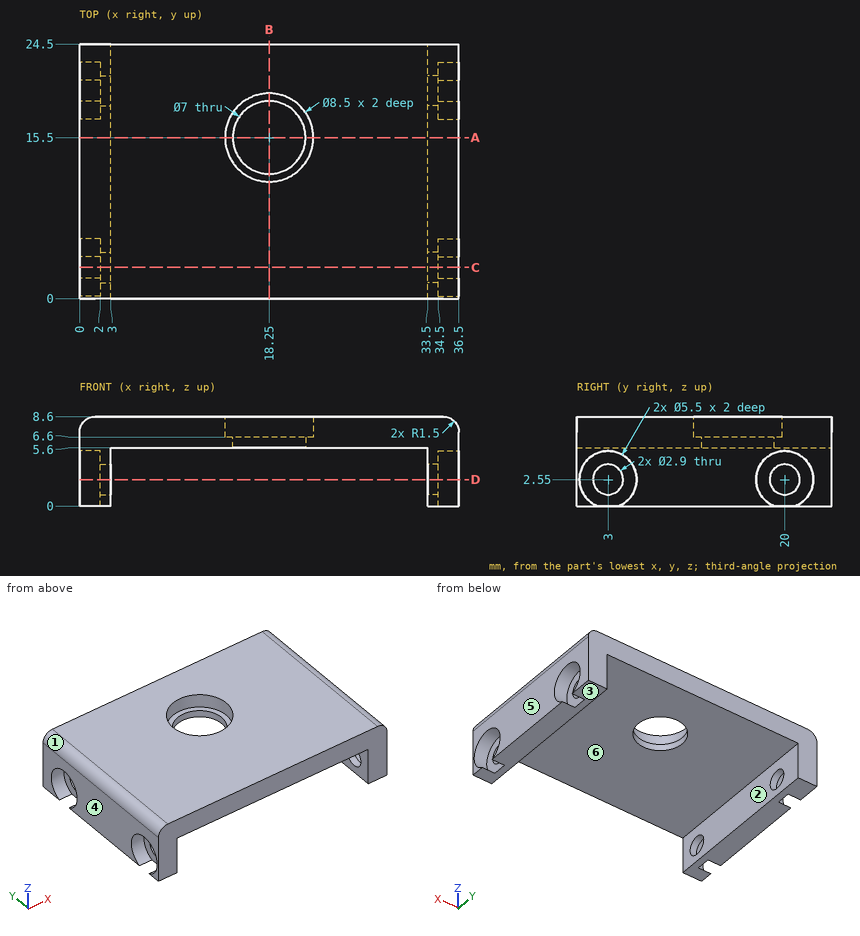
Source: three-view drawing plus pictorial views. Frame: mm from the lowest corner of the part. A direction names the side the tool comes from. Give positions to 0.01 mm unless a question says otherwise; leave off trailing zeros. Order: outer loops, then holes, each group sorted by start corner. A loop starts at its lowest first (then second) coordinate and runs counter-clockwise, first axis right, second up. Notation, with made-up numbers: M -18,-25 L 30,-25 A11 ccw 30,-19 Z; hole C 64.5,4.25 d1. An arc over 180 degrees is marked long. Return JSON: item names as keys, results as strings.
Item 1: Cut plane C-C (y = 3). Return loops of the section in (x, z), then the cut area to 3 significant figures.
Solutions:
{"outline": "M 0,5.3 L 2,5.3 L 2,4 L 3,4 L 3,5.6 L 33.5,5.6 L 33.5,4 L 34.5,4 L 34.5,5.3 L 36.5,5.3 L 36.5,7.1 A1.5 ccw 35,8.6 L 1.5,8.6 A1.5 ccw 0,7.1 Z; M 2,0 L 3,0 L 3,1.1 L 2,1.1 Z; M 33.5,0 L 34.5,0 L 34.5,1.1 L 33.5,1.1 Z", "area": "115 mm^2"}
Item 2: Cut plane A-A (y = 15.5). Return loops of the section in (x, z).
Solutions:
{"outline": "M 0,0 L 3,0 L 3,5.6 L 14.75,5.6 L 14.75,6.6 L 14,6.6 L 14,8.6 L 1.5,8.6 A1.5 ccw 0,7.1 Z; M 21.75,5.6 L 33.5,5.6 L 33.5,0 L 36.5,0 L 36.5,7.1 A1.5 ccw 35,8.6 L 22.5,8.6 L 22.5,6.6 L 21.75,6.6 Z"}
Item 3: Access query for the marked faces 1 and 2. Directions: +Z, -Z, +X, -X, +Y, -Y. A direction counts if a zero-diameter tool reaches every point of the face in a straight line with its end or side. Return the directions, or none.
Solutions:
{"face 1": "+Z, -X, +Y, -Y", "face 2": "-Z, +Y, -Y"}
Item 4: Cut plane B-B (x = 18.25). Return loops of the section in (y, z).
Solutions:
{"outline": "M 0,5.6 L 12,5.6 L 12,6.6 L 11.25,6.6 L 11.25,8.6 L 0,8.6 Z; M 19,5.6 L 24.5,5.6 L 24.5,8.6 L 19.75,8.6 L 19.75,6.6 L 19,6.6 Z"}
Item 5: Ray query, probe 1 along Y at (x, z) = (34.35, 2.55); probe 2 along Y at (x, z) = (35.65, 2.55); probe 3 along Y at (x, z) = (18.25, 6.3). Return the intervals inside material, ascending.
Solutions:
{"probe 1": "0 to 1.55, 4.45 to 18.55, 21.45 to 24.5", "probe 2": "0 to 0.25, 5.75 to 17.25, 22.75 to 24.5", "probe 3": "0 to 12, 19 to 24.5"}
Item 6: Cut plane D-D (z = 2.55). State how many separate pieces and enclosed holes the cut face has, then the cut area to 3 significant figures.
Solutions:
{"separate pieces": "6", "enclosed holes": "0", "area": "91.4 mm^2"}
Item 7: First-contact query: P1, Ø4, axis at y = 3, z = 2.55, coming from the +X side; P2, Ø7.5, axis at x = 16.5, y = 17.5, coming from the -Z side; P3, Ø1.6, axis at y = 20.5, z = 2, coming from the -X side; P4, Ø5.5, axis at x = 18.25, y = 15.5, coming from the -Z side. Flat tips, straight axial feed; report the tip coordinate or a pass-through.
Solutions:
{"P1": "x = 34.5", "P2": "z = 5.6", "P3": "x = 2", "P4": "through"}
Item 8: Pull-direction query (X, two-part tool) for the marked faces 3, 4, 5 and 6; classes: +X half, -X half, draft (parallel to the pull), parting line (faces both ways), or undercut.
Solutions:
{"face 3": "draft", "face 4": "-X half", "face 5": "+X half", "face 6": "undercut"}
